Design review of the part shown in the three views and the two pictorial views. Dimensions are in mm from the part's minimum x, y and z. Coordinates: 2 decimals unless noted, no trailing zeros. Write each loop counter-clockwise with the first axis right and the second up, starting at its lowest first coordinate (ties: lowest second). Pieces come first, ordered by that corner, then holes. Notation, with made-up numbers: (27, 84.25) -> (73, 84.25) arc R19 ccw to (73, 115.25) -> close; hole circle Ø7 at (88.25, 39.5). An arc over 180 degrees is marked (long way). Answer in a Markdown table with one row per item. Add a question column.
Item 1: Take a section at A-A, the plane z = 40.25. Write out the cut boundary in (x, y), and give its area (3 significant figures).
Item 2: Take a section at C-C, the plane z = 22.75. Write out the cut boundary in (x, y).
Item 3: Take a section at D-D, the plane z = 10. Write out the cut boundary in (x, y).
Item 4: Take a section at B-B, the plane x = 2.5. Write out the cut boundary in (y, z).
Item 5: To check wall thickness, follow line 1 (Y direction, x = 1.45, z = 5.25); line 2 (Z direction, x = 0.6, y = 70.5); line 3 (Y direction, x = 1.05, z = 23.5). State the ranges of each line that lie inside material, in increasing order.
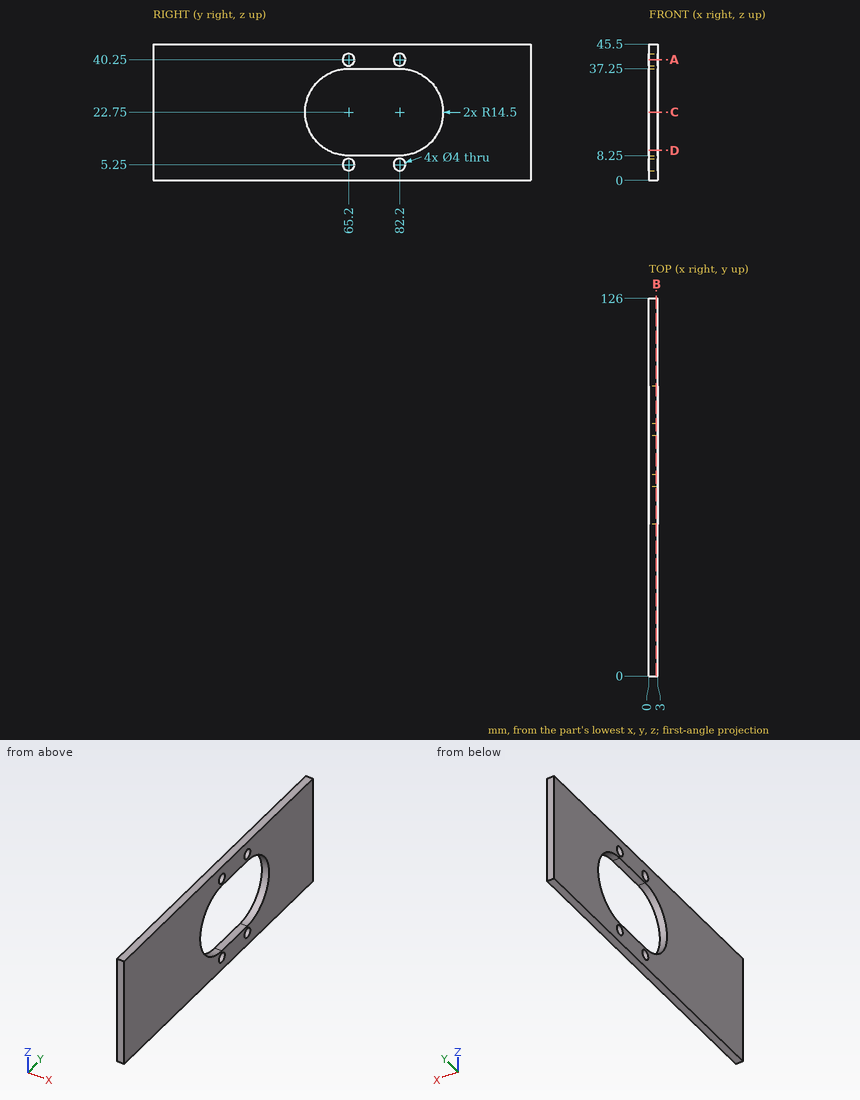
Answers:
| question | item | result |
|---|---|---|
| 1 | outline | (0, 0) -> (3, 0) -> (3, 63.2) -> (0, 63.2) -> close; (0, 67.2) -> (3, 67.2) -> (3, 80.2) -> (0, 80.2) -> close; (0, 84.2) -> (3, 84.2) -> (3, 126) -> (0, 126) -> close |
| 1 | area | 354 mm^2 |
| 2 | outline | (0, 0) -> (3, 0) -> (3, 50.7) -> (0, 50.7) -> close; (0, 96.7) -> (3, 96.7) -> (3, 126) -> (0, 126) -> close |
| 3 | outline | (0, 0) -> (3, 0) -> (3, 58.29) -> (0, 58.29) -> close; (0, 89.11) -> (3, 89.11) -> (3, 126) -> (0, 126) -> close |
| 4 | outline | (0, 0) -> (126, 0) -> (126, 45.5) -> (0, 45.5) -> close; hole circle Ø4 at (65.2, 5.25); hole circle Ø4 at (65.2, 40.25); hole (65.2, 8.25) -> (82.2, 8.25) arc R14.5 ccw to (82.2, 37.25) -> (65.2, 37.25) arc R14.5 ccw to start; hole circle Ø4 at (82.2, 5.25); hole circle Ø4 at (82.2, 40.25) |
| 5 | line 1 | y = 0 to 63.2, 67.2 to 80.2, 84.2 to 126 |
| 5 | line 2 | z = 0 to 8.25, 37.25 to 45.5 |
| 5 | line 3 | y = 0 to 50.72, 96.68 to 126 |
